Design review of the part built by this model. Coordinates are the model's own, in mm. Coordinates: 2 decimals unless noted, no trailing zeros. Loops run counter-clockwise (first coordinate to the right, second up) from the corner with the lowest first, then second, coordinate; pieces in that order, holes last. Notation, with made-up numbers: (9, -28.75) -> (35, -28.75) arc R17 cw to (35, -18.75) -> close; hole circle Ø2 at (-1.75, 37.25). An arc over 180 degrees is marked (long way). Answer as a JSON object with one key per item and string values.
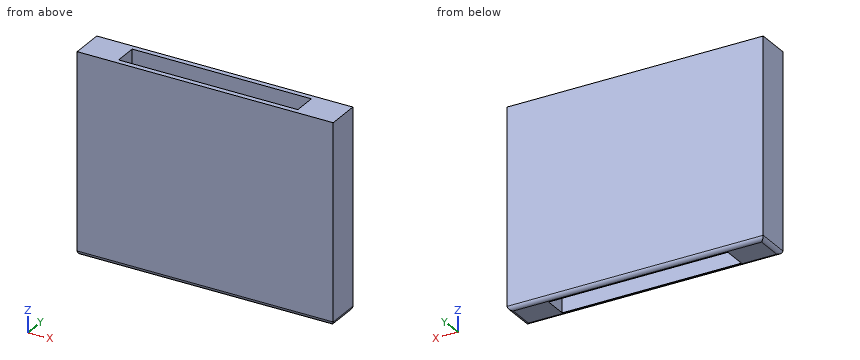
```python
from build123d import *

# Parameters (mm, degrees)
F0_W     = 50.8
F0_H     = 39.37
F1_DEPTH = 3.302
F2_W     = 35.56
F2_H     = 4.572
F3_DEPTH = 39.37
F4_R     = 0.762


with BuildPart() as f1:
    # F0 (on Front) → F1 (new body, symmetric)
    with BuildSketch(Plane.XZ):
        Rectangle(F0_W, F0_H)
    extrude(amount=F1_DEPTH, both=True)

    # F2 (on face) → F3 (cut)
    with BuildSketch(Plane.XY.offset(19.685)):
        Rectangle(F2_W, F2_H)
    extrude(amount=-F3_DEPTH, mode=Mode.SUBTRACT)

    # F4
    f4_edges = [f1.edges().sort_by_distance(p)[0] for p in [
        (0, -3.302, -19.685),
        (-25.4, 0, -19.685),
        (0, 3.302, -19.685),
        (25.4, 0, -19.685),
    ]]
    fillet(f4_edges, radius=F4_R)


solid = f1.part
```
1) Add section A-A, the plane x = -16. Give the boundary of the cut face in (y, z) (3 decimals), and give its area (3 significant figures).
Completed:
{"outline": "(-3.302, -18.923) arc R0.762 ccw to (-2.54, -19.685) -> (-2.286, -19.685) -> (-2.286, 19.685) -> (-3.302, 19.685) -> close; (2.286, -19.685) -> (2.54, -19.685) arc R0.762 ccw to (3.302, -18.923) -> (3.302, 19.685) -> (2.286, 19.685) -> close", "area": "79.8 mm²"}
2) Add section B-B, the plane z = -3.5. Give the boundary of the cut face in (x, y), and give its area (3 significant figures).
Completed:
{"outline": "(-25.4, -3.3) -> (25.4, -3.3) -> (25.4, 3.3) -> (-25.4, 3.3) -> close; hole (-17.78, -2.29) -> (17.78, -2.29) -> (17.78, 2.29) -> (-17.78, 2.29) -> close", "area": "173 mm²"}
3) Wall thickness on probe 1 along Y at (x, z) = (-2, -4.5); probe 2 along X at (y, z) = (-1.5, -12): over which ranges is each line inside the solid? List them lowest first.
Completed:
{"probe 1": "-3.3 to -2.29, 2.29 to 3.3", "probe 2": "-25.4 to -17.78, 17.78 to 25.4"}
4) Add section C-C, the plane y = -1. Give the boundary of the cut face in (x, z) (3 decimals).
Completed:
{"outline": "(-25.4, -18.923) arc R0.762 ccw to (-24.638, -19.685) -> (-17.78, -19.685) -> (-17.78, 19.685) -> (-25.4, 19.685) -> close; (17.78, -19.685) -> (24.638, -19.685) arc R0.762 ccw to (25.4, -18.923) -> (25.4, 19.685) -> (17.78, 19.685) -> close"}
